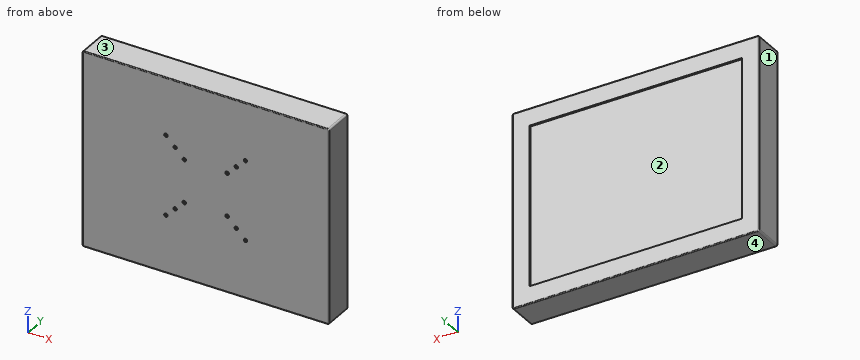
from build123d import *

# Parameters (mm, degrees)
SKETCH1_W           = 285
SKETCH1_H           = 225
BOSS_EXTRUDE1_DEPTH = 35
SKETCH2_W           = 245
SKETCH2_H           = 185
CUT_EXTRUDE1_DEPTH  = 2
FILLET1_R           = 2
FILLET2_R           = 1
FILLET3_R           = 1
SKETCH4_R           = 2
CUT_EXTRUDE2_DEPTH  = 2


with BuildPart() as part:
    # Sketch1 → Boss-Extrude1 (new body)
    with BuildSketch(Plane(origin=(0, 0, 0), x_dir=(1, 0, 0), z_dir=(0, 1, 0))):
        Rectangle(SKETCH1_W, SKETCH1_H)
    extrude(amount=BOSS_EXTRUDE1_DEPTH)

    # Sketch2 → Cut-Extrude1 (cut)
    with BuildSketch(Plane(origin=(0, 35, 0), x_dir=(1, 0, 0), z_dir=(0, 1, 0))):
        Rectangle(SKETCH2_W, SKETCH2_H)
    extrude(amount=-CUT_EXTRUDE1_DEPTH, mode=Mode.SUBTRACT)

    # Fillet1
    fillet1_edges = [part.edges().sort_by_distance(p)[0] for p in [
        (142.5, 17.5, 112.5),
        (-142.5, 17.5, 112.5),
        (-142.5, 17.5, -112.5),
        (142.5, 17.5, -112.5),
    ]]
    fillet(fillet1_edges, radius=FILLET1_R)

    # Fillet2
    fillet2_edges = [part.edges().sort_by_distance(p)[0] for p in [
        (-142.5, 35, 0),
        (0, 35, -112.5),
        (142.5, 35, 0),
        (0, 35, 112.5),
        (141.914213562, 35, 111.914213562),
        (141.914213562, 35, -111.914213562),
        (-141.914213562, 35, 111.914213562),
        (-141.914213562, 35, -111.914213562),
    ]]
    fillet(fillet2_edges, radius=FILLET2_R)

    # Fillet3
    fillet3_edges = [part.edges().sort_by_distance(p)[0] for p in [
        (-142.5, 0, 0),
        (142.5, 0, 0),
        (0, 0, 112.5),
        (0, 0, -112.5),
        (141.914213562, 0, 111.914213562),
        (141.914213562, 0, -111.914213562),
        (-141.914213562, 0, 111.914213562),
        (-141.914213562, 0, -111.914213562),
    ]]
    fillet(fillet3_edges, radius=FILLET3_R)

    # Sketch4 → Cut-Extrude2 (cut)
    with BuildSketch(Plane.XZ):
        with Locations((-24.748737342, 24.748737342)):
            Circle(SKETCH4_R)
        with Locations((-35.355339059, 35.355339059)):
            Circle(SKETCH4_R)
        with Locations((-45.961940777, 45.961940777)):
            Circle(SKETCH4_R)
        with Locations((24.748737342, 24.748737342)):
            Circle(SKETCH4_R)
        with Locations((35.355339059, 35.355339059)):
            Circle(SKETCH4_R)
        with Locations((45.961940777, 45.961940777)):
            Circle(SKETCH4_R)
        with Locations((24.748737342, -24.748737342)):
            Circle(SKETCH4_R)
        with Locations((35.355339059, -35.355339059)):
            Circle(SKETCH4_R)
        with Locations((45.961940777, -45.961940777)):
            Circle(SKETCH4_R)
        with Locations((-24.748737342, -24.748737342)):
            Circle(SKETCH4_R)
        with Locations((-35.355339059, -35.355339059)):
            Circle(SKETCH4_R)
        with Locations((-45.961940777, -45.961940777)):
            Circle(SKETCH4_R)
    extrude(amount=-CUT_EXTRUDE2_DEPTH, mode=Mode.SUBTRACT)


solid = part.part
Source: CAD feature listing. Evaluate the final solid. Frame: model axes, mm. Face numbers are marked on the shaded views. Coordinates: 2 decimals unless noted, no trailing zeros. Order: outer loops, then holes, each group sorted by start corner. A loop starts at its lowest first (then second) coordinate and runs counter-clockwise, first axis right, second up.
Item 1: Cut plane B-B (x = -16). Return loops of the section in (y, z), plus the area to 3 significant figures.
Output values:
outline: (0, -111.5) arc R1 ccw to (1, -112.5) - (34, -112.5) arc R1 ccw to (35, -111.5) - (35, -92.5) - (33, -92.5) - (33, 92.5) - (35, 92.5) - (35, 111.5) arc R1 ccw to (34, 112.5) - (1, 112.5) arc R1 ccw to (0, 111.5) - close
area: 7,500 mm2
Item 2: Pull-direction query (Z, two-part tool) for the marked faces 1, 2, 3 and 4; classes: pulls with the +Z half, pulls with the -Z half, needs draft (parallel to the pull), parting line crosses it, or undercut.
Output values:
face 1: needs draft
face 2: undercut
face 3: pulls with the +Z half
face 4: pulls with the -Z half
Item 3: Cut plane A-A (z = -84.5). Return loops of the section in (x, y).
Output values:
outline: (-142.5, 1) arc R1 ccw to (-141.5, 0) - (141.5, 0) arc R1 ccw to (142.5, 1) - (142.5, 34) arc R1 ccw to (141.5, 35) - (122.5, 35) - (122.5, 33) - (-122.5, 33) - (-122.5, 35) - (-141.5, 35) arc R1 ccw to (-142.5, 34) - close
Item 4: Material intervals for line 1 (Y direction, x = -49.5, z = 12), sorted ascending.
Output values:
line 1: y = 0 to 33
Item 5: First-contact query: P1, Ø3, axis at x = 45.96, z = 45.96, coming from the +Y side; P2, Ø3.5, axis at x = -45.96, z = -45.96, coming from the -Y side. Flat tips, straight axial feed; report the tip coordinate or a pass-through.
Output values:
P1: stops at y = 33
P2: stops at y = 2
